Read the model definition and answer for the solid it produces. Units are mm, in the model's axes. A direction names the side the tool comes from. Coordinates: 2 decimals unless noted, no trailing zeros. Write each loop counter-clockwise with the first axis right and the second up, starting at its lowest first coordinate (ties: lowest second). Pieces come first, ordered by that corner, then holes. Notation, with made-up numbers: (-6, -10) - (28, -10) arc R7 cw to (28, -5) - close; hole circle Ø7 at (7.25, 38.5). An arc over 180 degrees is marked (long way). Use a Markdown table: item, result.
from build123d import *

# Parameters (mm, degrees)
SKETCH1_W             = 711.2
SKETCH1_H             = 76.2
BOSS_EXTRUDE1_DEPTH   = 3.175
EDGE_FLANGE1_DEPTH    = 711.2
EDGE_FLANGE2_DEPTH    = 711.2
SKETCH14_R            = 2.667
UPPER_FLANGE_HP_DEPTH = 25.4
SKETCH16_R            = 3.3528
LOWER_FLANGE_HP_DEPTH = 717.03979687
LPATTERN1_COUNT       = 32
LPATTERN1_PITCH       = 25.4
SKETCH29_R            = 14.2875
CUT_EXTRUDE16_DEPTH   = 717.045619632
SKETCH31_W            = 35.56
SKETCH31_H            = 76.2
CUT_EXTRUDE11_DEPTH   = 716.954105561
SKETCH32_W            = 38.1
SKETCH32_H            = 76.2
CUT_EXTRUDE12_DEPTH   = 716.954105561
CUT_EXTRUDE13_START   = 217.547646287
CUT_EXTRUDE13_DEPTH   = 25.908
CUT_EXTRUDE13_START_2 = 467.744353713
CUT_EXTRUDE13_2_DEPTH = 25.908
SKETCH33_R            = 2.2479
SKETCH33_R_2          = 2.15
SKETCH33_R_3          = 2.24647347
SKETCH33_R_4          = 2.0193
CUT_EXTRUDE14_DEPTH   = 716.954105561


# Read off the part's stored shape, not the designer's step: Cut-Extrude13
# Sheet-metal steps are written as plain solids
with BuildPart() as part:
    # Sketch1 → Boss-Extrude1 (new body)
    with BuildSketch(Plane(origin=(0, 0, 0), x_dir=(1, 0, 0), z_dir=(0, 1, 0))):
        with Locations((355.6, 38.1)):
            Rectangle(SKETCH1_W, SKETCH1_H)
    extrude(amount=BOSS_EXTRUDE1_DEPTH)

    # Edge-Flange1 section (across the edge) → Edge-Flange1 (add)
    with BuildSketch(Plane(origin=(711.2, 0, 0.762), x_dir=(0, 0, -1), z_dir=(-1, 0, 0))):
        with BuildLine():
            Line((-3.175, 0.762), (-3.175, 15.875))
            Line((-3.175, 15.875), (0, 15.875))
            Line((0, 15.875), (0, 0.762))
            ThreePointArc((0, 0.762), (0.223184633, 0.223184633), (0.762, 0))
            Line((0.762, 0), (0.762, -3.175))
            ThreePointArc((0.762, -3.175), (-2.021879398, -2.021879398), (-3.175, 0.762))
        make_face()
    extrude(amount=EDGE_FLANGE1_DEPTH)

    # Edge-Flange2 section (across the edge) → Edge-Flange2 (add)
    with BuildSketch(Plane(origin=(0, 0, -76.962), x_dir=(0, 0, 1), z_dir=(1, 0, 0))):
        with BuildLine():
            Line((-3.175, 0.762), (-3.175, 19.05))
            Line((-3.175, 19.05), (0, 19.05))
            Line((0, 19.05), (0, 0.762))
            ThreePointArc((0, 0.762), (0.223184633, 0.223184633), (0.762, 0))
            Line((0.762, 0), (0.762, -3.175))
            ThreePointArc((0.762, -3.175), (-2.021879398, -2.021879398), (-3.175, 0.762))
        make_face()
    extrude(amount=EDGE_FLANGE2_DEPTH)

    # Sketch14 → upper flange HP (cut)
    with BuildSketch(Plane(origin=(0, 0, -80.137), x_dir=(-1, 0, 0), z_dir=(0, 0, -1))):
        with Locations(Location((-12.7, -12.7, 0), (0, 0, 90))):
            Circle(SKETCH14_R)
        with Locations(Location((-38.1, -12.7, 0), (0, 0, 90))):
            Circle(SKETCH14_R)
        with Locations(Location((-63.5, -12.7, 0), (0, 0, 90))):
            Circle(SKETCH14_R)
        with Locations(Location((-88.9, -12.7, 0), (0, 0, 90))):
            Circle(SKETCH14_R)
        with Locations(Location((-114.3, -12.7, 0), (0, 0, 90))):
            Circle(SKETCH14_R)
        with Locations(Location((-139.7, -12.7, 0), (0, 0, 90))):
            Circle(SKETCH14_R)
        with Locations(Location((-165.1, -12.7, 0), (0, 0, 90))):
            Circle(SKETCH14_R)
        with Locations(Location((-190.5, -12.7, 0), (0, 0, 90))):
            Circle(SKETCH14_R)
        with Locations(Location((-215.9, -12.7, 0), (0, 0, 90))):
            Circle(SKETCH14_R)
        with Locations(Location((-241.3, -12.7, 0), (0, 0, 90))):
            Circle(SKETCH14_R)
        with Locations(Location((-266.7, -12.7, 0), (0, 0, 90))):
            Circle(SKETCH14_R)
        with Locations(Location((-292.1, -12.7, 0), (0, 0, 90))):
            Circle(SKETCH14_R)
        with Locations(Location((-317.5, -12.7, 0), (0, 0, 90))):
            Circle(SKETCH14_R)
        with Locations(Location((-342.9, -12.7, 0), (0, 0, 90))):
            Circle(SKETCH14_R)
        with Locations(Location((-368.3, -12.7, 0), (0, 0, 90))):
            Circle(SKETCH14_R)
        with Locations(Location((-393.7, -12.7, 0), (0, 0, 90))):
            Circle(SKETCH14_R)
        with Locations(Location((-419.1, -12.7, 0), (0, 0, 90))):
            Circle(SKETCH14_R)
        with Locations(Location((-444.5, -12.7, 0), (0, 0, 90))):
            Circle(SKETCH14_R)
        with Locations(Location((-469.9, -12.7, 0), (0, 0, 90))):
            Circle(SKETCH14_R)
        with Locations(Location((-495.3, -12.7, 0), (0, 0, 90))):
            Circle(SKETCH14_R)
        with Locations(Location((-520.7, -12.7, 0), (0, 0, 90))):
            Circle(SKETCH14_R)
        with Locations(Location((-546.1, -12.7, 0), (0, 0, 90))):
            Circle(SKETCH14_R)
        with Locations(Location((-571.5, -12.7, 0), (0, 0, 90))):
            Circle(SKETCH14_R)
        with Locations(Location((-596.9, -12.7, 0), (0, 0, 90))):
            Circle(SKETCH14_R)
        with Locations(Location((-622.3, -12.7, 0), (0, 0, 90))):
            Circle(SKETCH14_R)
        with Locations(Location((-647.7, -12.7, 0), (0, 0, 90))):
            Circle(SKETCH14_R)
        with Locations(Location((-673.1, -12.7, 0), (0, 0, 90))):
            Circle(SKETCH14_R)
        with Locations(Location((-698.5, -12.7, 0), (0, 0, 90))):
            Circle(SKETCH14_R)
        with Locations((-723.9, -12.7)):
            Circle(SKETCH14_R)
        with Locations((-749.3, -12.7)):
            Circle(SKETCH14_R)
        with Locations((-774.7, -12.7)):
            Circle(SKETCH14_R)
        with Locations((-800.1, -12.7)):
            Circle(SKETCH14_R)
    extrude(amount=-UPPER_FLANGE_HP_DEPTH, mode=Mode.SUBTRACT)

    # Sketch16 → Lower flange HP (cut, through all)
    with BuildSketch(Plane(origin=(0, 0, 0.762), x_dir=(-1, 0, 0), z_dir=(0, 0, -1))):
        with Locations(Location((-698.5, -9.525, 0), (0, 0, 90))):
            Circle(SKETCH16_R)
    lower_flange_hp = extrude(amount=-LOWER_FLANGE_HP_DEPTH, mode=Mode.SUBTRACT)

    # LPattern1: Lower flange HP ×32
    with Locations(*[(-i * LPATTERN1_PITCH, 0, 0) for i in range(1, LPATTERN1_COUNT)]):
        add(lower_flange_hp, mode=Mode.SUBTRACT)

    # Sketch29 → Cut-Extrude16 (cut, through all)
    with BuildSketch(Plane(origin=(0, 3.175, 0), x_dir=(1, 0, 0), z_dir=(0, 1, 0))):
        with Locations(Location((584.2, 38.1, 0), (0, 0, 270))):
            Circle(SKETCH29_R)
        with Locations(Location((127, 38.1, 0), (0, 0, 270))):
            Circle(SKETCH29_R)
    extrude(amount=-CUT_EXTRUDE16_DEPTH, mode=Mode.SUBTRACT)

    # Sketch31 → Cut-Extrude11 (cut, through all)
    with BuildSketch(Plane.XZ):
        with Locations((693.42, -38.1)):
            Rectangle(SKETCH31_W, SKETCH31_H)
    extrude(amount=-CUT_EXTRUDE11_DEPTH, mode=Mode.SUBTRACT)

    # Sketch32 → Cut-Extrude12 (cut, through all)
    with BuildSketch(Plane.XZ):
        with Locations((19.05, -38.1)):
            Rectangle(SKETCH32_W, SKETCH32_H)
    extrude(amount=-CUT_EXTRUDE12_DEPTH, mode=Mode.SUBTRACT)

    # Cut-Extrude13 outline → Cut-Extrude13 (cut)
    with BuildSketch(Plane.YZ.offset(CUT_EXTRUDE13_START)):
        with BuildLine():
            Line((3.175, -76.2), (3.175, -51.054))
            Line((3.175, -51.054), (0, -51.054))
            Line((0, -51.054), (0, -76.2))
            ThreePointArc((0, -76.2), (-0.003610771, -76.274093029), (-0.014408863, -76.347483871))
            Line((-0.014408863, -76.347483871), (3.100554207, -76.962))
            ThreePointArc((3.100554207, -76.962), (3.156344352, -76.582813981), (3.175, -76.2))
        make_face()
    extrude(amount=CUT_EXTRUDE13_DEPTH, mode=Mode.SUBTRACT)

    # Cut-Extrude13 2 outline → Cut-Extrude13 2 (cut)
    with BuildSketch(Plane.YZ.offset(CUT_EXTRUDE13_START_2)):
        with BuildLine():
            Line((3.175, -76.2), (3.175, -51.054))
            Line((3.175, -51.054), (0, -51.054))
            Line((0, -51.054), (0, -76.2))
            ThreePointArc((0, -76.2), (-0.003610771, -76.274093029), (-0.014408863, -76.347483871))
            Line((-0.014408863, -76.347483871), (3.100554207, -76.962))
            ThreePointArc((3.100554207, -76.962), (3.156344352, -76.582813981), (3.175, -76.2))
        make_face()
    extrude(amount=CUT_EXTRUDE13_2_DEPTH, mode=Mode.SUBTRACT)

    # Sketch33 → Cut-Extrude14 (cut, through all)
    with BuildSketch(Plane(origin=(0, 0, 0), x_dir=(-1, 0, 0), z_dir=(0, -1, 0))):
        with Locations(Location((-109.5127, 56.848002955, 0), (0, 0, 270))):
            Circle(SKETCH33_R)
        with Locations(Location((-144.973212242, 57.308515197, 0), (0, 0, 270))):
            Circle(SKETCH33_R_2)
        with Locations(Location((-144.5127, 21.848002955, 0), (0, 0, 270))):
            Circle(SKETCH33_R_3)
        with Locations(Location((-109.052187758, 21.387490713, 0), (0, 0, 270))):
            Circle(SKETCH33_R_4)
        with Locations(Location((-602.147812242, 21.387490713, 0), (0, 0, 90))):
            Circle(SKETCH33_R_4)
        with Locations(Location((-566.6873, 21.848002955, 0), (0, 0, 90))):
            Circle(SKETCH33_R_3)
        with Locations(Location((-566.226787758, 57.308515197, 0), (0, 0, 90))):
            Circle(SKETCH33_R_2)
        with Locations(Location((-601.6873, 56.848002955, 0), (0, 0, 90))):
            Circle(SKETCH33_R)
    extrude(amount=-CUT_EXTRUDE14_DEPTH, mode=Mode.SUBTRACT)


solid = part.part
(1) Each of these flat-tipped pins is pushed along its axis until it touches: P1, Ø3, axis at x = 602.15, z = -21.39, coming from the -Y side; P2, Ø12, axis at x = 579, z = -60.5, coming from the -Y side; P3, Ø5, axis at x = 393.7, y = -12.7, coming from the -Z side; P4, Ø6, axis at x = 622.3, y = -9.525, coming from the +Z side. Where does it stop, or does it pass through?
Report:
| item | result |
|---|---|
| P1 | passes through |
| P2 | stops at y = 0 |
| P3 | stops at z = 0.76 |
| P4 | stops at z = -76.96 |
(2) For faces 1 (the flat face through (361, -8, 3.937)), 2 (the flat face through (361, -8, 0.762)), determine the directions among +Z, -Z, +X, -X, +Y, -Y from which every point of the face is accessible in a straight line to the end or side of a thin tool.
Report:
| item | result |
|---|---|
| face 1 | +Z, +X, -X, +Y, -Y |
| face 2 | +X, -X, -Y |
(3) Straight lines are drawn through the part: L1, parallel to Z at x = 209, y = -2.75; L2, parallel to X at y = 1.15, z = -38.1; L3, parallel to Y at x = 404, z = -60 (3 decimals). For each, find the intervals that lie inside material, in ascending order.
Report:
| item | result |
|---|---|
| L1 | z = -80.14 to -76.96, 0.76 to 3.94 |
| L2 | x = 38.1 to 112.71, 141.29 to 569.91, 598.49 to 675.64 |
| L3 | y = 0 to 3.175 |
(4) The mould has two halves that part along X. Classify faces 3 (the flat face through (351, -10, -76.962)), 4 (the cylindrical face through (598.366, 1.61, -39.96)): pulls with the +X half, pulls with the -X half, needs draft (parallel to the pull), parting line crosses it, or undercut.
Report:
| item | result |
|---|---|
| face 3 | needs draft |
| face 4 | undercut |
(5) A cutting plane is placed at B-B, the plane x = 530. Write down the section's boundary in (y, z) (3 decimals).
Report:
| item | result |
|---|---|
| outline | (-19.05, -80.137) - (-0.762, -80.137) arc R3.937 ccw to (3.175, -76.2) - (3.175, 0) arc R3.937 ccw to (-0.762, 3.937) - (-15.875, 3.937) - (-15.875, 0.762) - (-0.762, 0.762) arc R0.762 cw to (0, 0) - (0, -76.2) arc R0.762 cw to (-0.762, -76.962) - (-19.05, -76.962) - close |
(6) A cutting plane is placed at A-A, the plane z = -38.1. Write down the section's boundary in (x, y) (1 decimal).
Report:
| item | result |
|---|---|
| outline | (38.1, 0) - (112.7, 0) - (112.7, 3.2) - (38.1, 3.2) - close; (141.3, 0) - (569.9, 0) - (569.9, 3.2) - (141.3, 3.2) - close; (598.5, 0) - (675.6, 0) - (675.6, 3.2) - (598.5, 3.2) - close |
